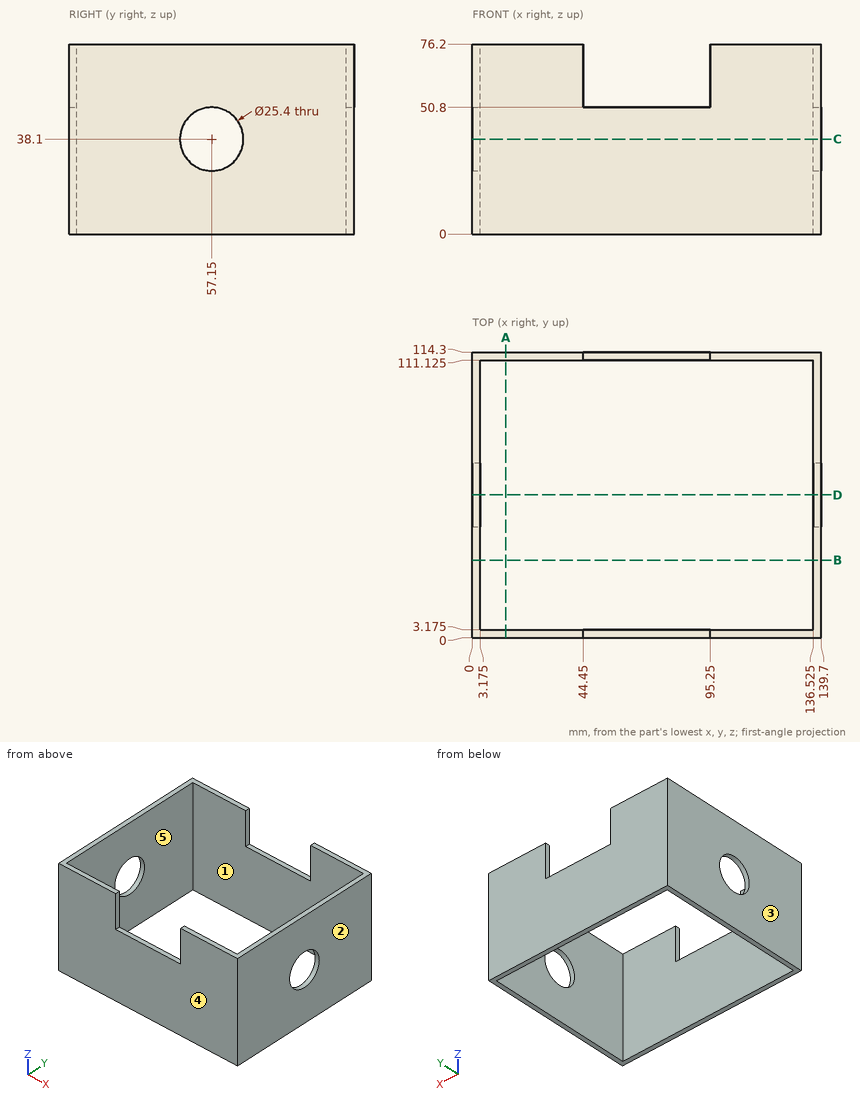
Verification items for this drawing (mm, ordinates from the low corner). A direction names the side the tool comes from. Coordinates: 2 decimals unless noted, no trailing zeros. Write each loop counter-clockwise with the first axis right and the second up, starting at its lowest first coordinate (ties: lowest second). Pieces come first, ordered by that corner, then holes. Notation, with made-up numbers: M 29,1 L 86,1 A22 cw 86,16 Z; hole C 77,45 d1. An arc over 180 degrees is marked long. Use one line per item in the form item = value. Start each with the question number.
1) Thickness scan on probe 1 along X at (y, z) = (93.5, 8.5) (3 decimals); probe 2 along Y at (x, z) = (112, 28) (3 decimals); probe 3 along Y at (x, z) = (137, 38). Record the ranges inside material, lowest first. Write a range as from..to.
2) Section check A-A on x = 13.5. Enter the section's corners in (y, z) (3 decimals), and give its area (3 significant figures).
3) Section check C-C on z = 38.1. Enter the section's corners in (x, y) (3 decimals).
4) Release check for a two-part mould opening along Y. For the marked faces 3, 4 and 5 record: pulls with the +Y half, pulls with the -Y half, needs draft (parallel to the pull), parting line crosses it, or undercut.
5) Set-up check for the marked faces 1 and 2: record each of +Z, -Z, +X, -X, +Y, -Y from which the full face is reachable in a straight line by a thin tool's end or side.
6) Section check D-D on y = 57.15. Enter the section's corners in (x, z) (3 decimals), and give its area (3 significant figures).
7) Section check B-B on y = 31. Enter the section's corners in (x, z) (3 decimals), and give its area (3 significant figures).
8) Go/stop test with flat-tipped pins: pin 1 Ø15 at (y, z) = (57.15, 38.1) entering from +X; pin 2 Ø3.5 at (x, y) = (72, 112.5) entering from +Z. Record where each tip stops, or that it passes through.
Responses:
q1.probe_1 = 0..3.175, 136.525..139.7
q1.probe_2 = 0..3.175, 111.125..114.3
q1.probe_3 = 0..44.45, 69.85..114.3
q2.outline = M 0,0 L 3.175,0 L 3.175,76.2 L 0,76.2 Z; M 111.125,0 L 114.3,0 L 114.3,76.2 L 111.125,76.2 Z
q2.area = 484 mm2
q3.outline = M 0,0 L 139.7,0 L 139.7,44.45 L 136.525,44.45 L 136.525,3.175 L 3.175,3.175 L 3.175,44.45 L 0,44.45 Z; M 0,69.85 L 3.175,69.85 L 3.175,111.125 L 136.525,111.125 L 136.525,69.85 L 139.7,69.85 L 139.7,114.3 L 0,114.3 Z
q4.face_3 = needs draft
q4.face_4 = pulls with the -Y half
q4.face_5 = undercut
q5.face_1 = +Z, -Z
q5.face_2 = +Z, -Z, +X, +Y, -Y
q6.outline = M 0,0 L 3.175,0 L 3.175,25.4 L 0,25.4 Z; M 0,50.8 L 3.175,50.8 L 3.175,76.2 L 0,76.2 Z; M 136.525,0 L 139.7,0 L 139.7,25.4 L 136.525,25.4 Z; M 136.525,50.8 L 139.7,50.8 L 139.7,76.2 L 136.525,76.2 Z
q6.area = 323 mm2
q7.outline = M 0,0 L 3.175,0 L 3.175,76.2 L 0,76.2 Z; M 136.525,0 L 139.7,0 L 139.7,76.2 L 136.525,76.2 Z
q7.area = 484 mm2
q8.pin_1 = through
q8.pin_2 = 50.8
